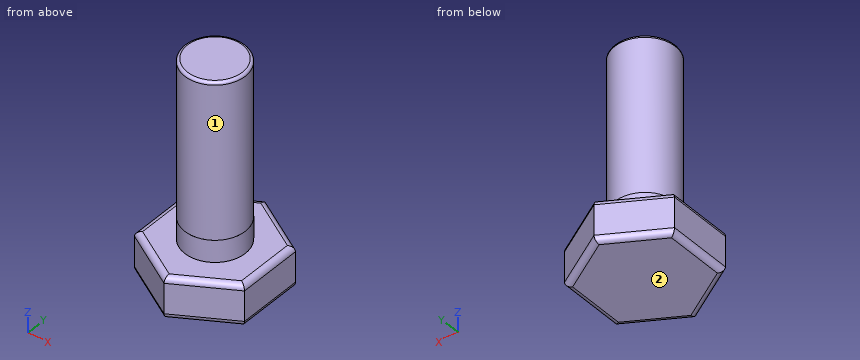
```python
from build123d import *

# Parameters (mm, degrees)
EXTRUDE_437_DEPTH = 15
SKETCH_2_R        = 11
EXTRUDE_1_DEPTH   = 8
FILLET_3_R        = 2
SKETCH_3_R        = 10.995
EXTRUDE_1_2_DEPTH = 57
FILLET_4_R        = 1


with BuildPart() as part:
    # 草图1 → Extrude 437 (new body)
    with BuildSketch(Plane.XY):
        Polygon((20, 11.547005384), (0, 23.094010768), (-20, 11.547005384), (-20, -11.547005384), (0, -23.094010768), (20, -11.547005384), align=None)
    extrude(amount=EXTRUDE_437_DEPTH)

    # 草图2 → Extrude 1 (add)
    with BuildSketch(Plane.XY.offset(15)):
        Circle(SKETCH_2_R)
    extrude(amount=EXTRUDE_1_DEPTH)

    # 圆角3
    fillet_3_edges = [part.edges().sort_by_distance(p)[0] for p in [
        (-10, 17.320508076, 15),
        (-20, 0, 15),
        (-10, -17.320508076, 15),
        (10, -17.320508076, 15),
        (20, 0, 15),
        (10, -17.320508076, 0),
        (-10, -17.320508076, 0),
        (-20, 0, 0),
        (10, 17.320508076, 15),
        (-10, 17.320508076, 0),
        (10, 17.320508076, 0),
        (20, 0, 0),
    ]]
    fillet(fillet_3_edges, radius=FILLET_3_R)

    # 草图3 → Extrude 1 2 (add)
    with BuildSketch(Plane.XY.offset(23)):
        Circle(SKETCH_3_R)
    extrude(amount=EXTRUDE_1_2_DEPTH)

    # 圆角4
    fillet_4_edges = [part.edges().sort_by_distance(p)[0] for p in [
        (-10.995, 0, 80),
    ]]
    fillet(fillet_4_edges, radius=FILLET_4_R)


solid = part.part
```
Model file for the job. Use its own axes, mm. Face numbers are marked on the shaded views. A direction names the side the tool comes from. Round coordinates to 2 decimals unless told otherwise and drop trailing zeros. Write each loop counter-clockwise with the first axis right and the second up, starting at its lowest first coordinate (ties: lowest second). Pieces come first, ordered by that corner, then holes. Notation, with made-up numbers: (74.5, -1) -> (78.5, -1) arc R10 ccw to (78.5, 12) -> close; hole circle Ø4 at (57, 59). An arc over 180 degrees is marked (long way). Answer as CSV lines item,"result".
1. Slice it at A-A, the plane y = 0. List the corners of the cut face in (x, z) (3 decimals), plus the area to 3 significant figures.
Resolved:
outline,"(-20, 2) arc R2 ccw to (-18, 0) -> (18, 0) arc R2 ccw to (20, 2) -> (20, 13) arc R2 ccw to (18, 15) -> (11, 15) -> (11, 23) -> (10.995, 23) -> (10.995, 79) arc R1 ccw to (9.995, 80) -> (-9.995, 80) arc R1 ccw to (-10.995, 79) -> (-10.995, 23) -> (-11, 23) -> (-11, 15) -> (-18, 15) arc R2 ccw to (-20, 13) -> close"
area,"2,030 mm²"
2. Slice it at C-C, the plane z = 58.5. List the corners of the cut face in (x, y) (3 decimals), plus the area to 3 significant figures.
Resolved:
outline,"circle Ø21.99 at (0, 0)"
area,"380 mm²"
3. Pin check, flat tips, straight feed: pin 1 Ø1 at (x, y) = (7, 10) entering from +Z; pin 2 Ø1 at (x, z) = (2, 68) entering from +Y; pin 3 Ø5 at (y, z) = (-11.5, 61.5) entering from +X. Stop position of each tip, or through.
Resolved:
pin 1,"z = 15"
pin 2,"y = 10.89"
pin 3,"x = 6.32"
4. Slice it at D-D, the plane z = 21. List the corners of the cut face in (x, y).
Resolved:
outline,"circle Ø22 at (0, 0)"
5. Drill centre lines: line 1 (Z direction, x = -7.5, y = -14.5); line 2 (X direction, y = -4, z = 59.5); line 3 (Y direction, x = -8, z = 18.5). Where is each one in solid material? Low to high.
Resolved:
line 1,"0 to 15"
line 2,"-10.24 to 10.24"
line 3,"-7.55 to 7.55"
6. Slice it at B-B, the plane z = 10. List the corners of the cut face in (x, y), plus the area to 3 significant figures.
Resolved:
outline,"(-20, -11.55) -> (0, -23.09) -> (20, -11.55) -> (20, 11.55) -> (0, 23.09) -> (-20, 11.55) -> close"
area,"1,390 mm²"
7. Tool access for the marked faces 1 and 2: list every direction of +Z, -Z, +X, -X, +Y, -Y with a clear straight run to the whole face (end or side of a thin tool).
Resolved:
face 1,"+Z"
face 2,"-Z, +X, -X, +Y, -Y"
